from build123d import *

# Parameters (mm, degrees)
F0_R     = 3.3798618289
F0_R_2   = 1.5875
F1_DEPTH = 30.48


with BuildPart() as f1:
    # F0 (on Front) → F1 (new body)
    with BuildSketch(Plane.XZ):
        with BuildLine():
            ThreePointArc((-3.1763056217, 0), (0, 3.1763056217), (3.1763056217, 0))
            Line((3.1763056217, 0), (7.9375, 0))
            ThreePointArc((7.9375, 0), (0, 7.9375), (-7.9375, 0))
            Line((-7.9375, 0), (-3.1763056217, 0))
        make_face()
        with BuildLine():
            Line((7.9375, 0), (3.1763056217, 0))
            ThreePointArc((3.1763056217, 0), (0, -3.1763056217), (-3.1763056217, 0))
            Line((-3.1763056217, 0), (-7.9375, 0))
            ThreePointArc((-7.9375, 0), (-5.6126600757, -5.6126600757), (0, -7.9375))
            ThreePointArc((0, -7.9375), (5.6126600757, -5.6126600757), (7.9375, 0))
        make_face()
        with BuildLine():
            ThreePointArc((-7.9375, 0), (0, 7.9375), (7.9375, 0))
            Line((7.9375, 0), (36.5125, 0))
            ThreePointArc((36.5125, 0), (38.8373399243, 5.6126600757), (44.45, 7.9375))
            Line((44.45, 7.9375), (18.003602441, 7.9375))
            ThreePointArc((18.003602441, 7.9375), (12.0425977283, 10.6272719893), (10.1151377075, 16.876539819))
            Line((10.1151377075, 16.876539819), (15.5735553324, 60.4210392487))
            ThreePointArc((15.5735553324, 60.4210392487), (0.1766226081, 47.6259825673), (-15.5011920437, 60.0752853808))
            Line((-15.5011920437, 60.0752853808), (-7.9375, 0))
        make_face()
        with BuildLine():
            Line((36.5125, 0), (7.9375, 0))
            ThreePointArc((7.9375, 0), (5.6126600757, -5.6126600757), (0, -7.9375))
            Line((0, -7.9375), (44.45, -7.9375))
            ThreePointArc((44.45, -7.9375), (38.8373399243, -5.6126600757), (36.5125, 0))
        make_face()
        with BuildLine():
            ThreePointArc((44.45, 7.9375), (38.8373399243, 5.6126600757), (36.5125, 0))
            ThreePointArc((36.5125, 0), (38.8373399243, -5.6126600757), (44.45, -7.9375))
            ThreePointArc((44.45, -7.9375), (50.0626600757, -5.6126600757), (52.3875, 0))
            ThreePointArc((52.3875, 0), (50.0626600757, 5.6126600757), (44.45, 7.9375))
        make_face()
        with BuildLine():
            ThreePointArc((47.3488403966, 0), (44.45, -2.8988403966), (41.5511596034, 0))
            ThreePointArc((41.5511596034, 0), (44.45, 2.8988403966), (47.3488403966, 0))
        make_face(mode=Mode.SUBTRACT)
        with BuildLine():
            ThreePointArc((-15.7474550599, 65.5083037958), (-15.8587171211, 62.7811702055), (-15.5011920437, 60.0752853808))
            ThreePointArc((-15.5011920437, 60.0752853808), (0.1766226081, 47.6259825673), (15.5735553324, 60.4210392487))
            ThreePointArc((15.5735553324, 60.4210392487), (15.7994591031, 61.9531590098), (15.875, 63.5))
            Line((15.875, 63.5), (15.3865317539, 67.407718719))
            ThreePointArc((15.3865317539, 67.407718719), (-0.9667009211, 79.3455392565), (-15.7474550599, 65.5083037958))
        make_face()
        with Locations((0, 63.5)):
            Circle(F0_R, mode=Mode.SUBTRACT)
        with BuildLine():
            Line((-9.5249557191, 114.3), (-15.7474550599, 65.5083037958))
            ThreePointArc((-15.7474550599, 65.5083037958), (-0.9667009211, 79.3455392565), (15.3865317539, 67.407718719))
            Line((15.3865317539, 67.407718719), (9.5249557191, 114.3))
            ThreePointArc((9.5249557191, 114.3), (9.5249889298, 114.2854780636), (9.525, 114.2709560934))
            ThreePointArc((9.525, 114.2709560934), (-0.0145219702, 104.7459671636), (-9.5249557191, 114.3))
        make_face()
        with Locations((-6.1838091351, 100.0252)):
            Circle(F0_R_2, mode=Mode.SUBTRACT)
        with BuildLine():
            Line((15.3865317539, 67.407718719), (15.875, 63.5))
            ThreePointArc((15.875, 63.5), (15.7524096029, 65.4690649313), (15.3865317539, 67.407718719))
        make_face()
        with BuildLine():
            ThreePointArc((9.5249557191, 114.3), (0, 123.7959560934), (-9.5249557191, 114.3))
            ThreePointArc((-9.5249557191, 114.3), (-0.0145219702, 104.7459671636), (9.525, 114.2709560934))
            ThreePointArc((9.525, 114.2709560934), (9.5249889298, 114.2854780636), (9.5249557191, 114.3))
        make_face()
        with BuildLine():
            ThreePointArc((3.175, 114.2709560934), (-0.0048406567, 111.0959597835), (-3.1749852397, 114.2806373956))
            ThreePointArc((-3.1749852397, 114.2806373956), (0.0048406567, 117.4459524033), (3.175, 114.2709560934))
        make_face(mode=Mode.SUBTRACT)
    extrude(amount=-F1_DEPTH)


solid = f1.part
Design review of the part built by this model. Coordinates are the model's own, in mm. A direction names the side the tool comes from. Give positions to 0.01 mm unless a question says otherwise; leave off trailing zeros. Loops run counter-clockwise (first coordinate to the right, second up) from the corner with the lowest first, then second, coordinate; pieces in that order, holes last. Notation, with made-up numbers: (9.25, 20) - (13.25, 20) arc R11 ccw to (13.25, 40) - close; hole circle Ø6 at (59, -3). An arc over 180 degrees is marked (long way). Use CSV: the item, a comma, the result in double quotes. Start each with the question number.
1. Machinability: for faces 4 (the flat face through (22, 15, -7.938)), 5 (the flat face through (31, 15, 7.938)), which of the approach directions +Z, -Z, +X, -X, +Y, -Y give a long, thin tool a straight path to every point of the face, cutting with its end or side? Answer none if there is none.
2. Wall thickness on L1, parallel to Z at x = 0, y = 8; L2, parallel to Z at x = 35, y = 8; L3, parallel to X at y = 23, z = 63: over which ranges is each line inside the solid? List them lowest first.
3. Add section D-D (z = 43). State the section outline as (x, y) points, plus the area to 3 significant figures.
4. Add section C-C (x = 28). State the section outline as (y, z) points.
5. Add section A-A (z = 1.5). State the section outline as (x, y) points, plus the area to 3 significant figures.
6. Insertion check: P1, Ø5, axis at y = 13.5, z = 26.5, coming from the +X side; P2, Ø3, axis at x = 39, y = 13, coming from the +Z side; P3, Ø2, axis at x = -3.5, y = 17, coming from the +Z side. Each pin has a flat end and moves straight along its axis. Give the tip position at first contact, or say it passes through.
7. Add section B-B (y = 7). Count the separate pieces of the cut face and the enclosed holes in it, plus the area to 3 significant figures.
8. Draft analysis for pull direction X (two halves, no side actions). For faces 1 (the flat face through (12.8, 15, 38.3)), 2 (the cylindrical face through (-0.44, 15.03, 66.85)), 3 (the cylindrical face through (0.209, 15.027, 123.794)), state which applies: released by +X, released by -X, zero draft, split by the parting line, or undercut.
Results found:
1,face 4,"-Z, +X, -X, +Y, -Y"
1,face 5,"+Z, +X, +Y, -Y"
2,L1,"z = -7.94 to -3.18, 3.18 to 60.12, 66.88 to 111.1, 117.45 to 123.8"
2,L2,"z = -7.94 to 7.94"
2,L3,"x = -15.87 to -3.34, 3.34 to 15.87"
3,outline,"(-13.35, 0) - (13.39, 0) - (13.39, 30.48) - (-13.35, 30.48) - close"
3,area,"815 mm²"
4,outline,"(0, -7.94) - (30.48, -7.94) - (30.48, 7.94) - (0, 7.94) - close"
5,outline,"(-8.13, 0) - (-2.8, 0) - (-2.8, 30.48) - (-8.13, 30.48) - close; (2.8, 0) - (41.97, 0) - (41.97, 30.48) - (2.8, 30.48) - close; (46.93, 0) - (52.24, 0) - (52.24, 30.48) - (46.93, 30.48) - close"
5,area,"1,520 mm²"
6,P1,"stops at x = 11.63"
6,P2,"stops at z = 7.94"
6,P3,"stops at z = 123.46"
7,separate pieces,"1"
7,enclosed holes,"5"
7,area,"3,630 mm²"
8,face 1,"released by +X"
8,face 2,"undercut"
8,face 3,"split by the parting line"
